Read the model definition and answer for the solid it produces. Units are mm, in the model's axes. A direction names the side the tool comes from. Coordinates: 2 decimals unless noted, no trailing zeros. Write each loop counter-clockwise with the first axis right and the second up, starting at its lowest first coordinate (ties: lowest second). Pieces come first, ordered by that corner, then holes.
1) The part is cut by section B-B (x = 0). Determine the outline of the cut face in (y, z), then the cut area to 3 significant figures.
2) The part is cut by section A-A (z = 0). Determine the outline of the cut face in (x, y), then the cut area to 3 significant figures.
3) Which of the six approach directions +Z, -Z, +X, -X, +Y, -Y give full straight-line access (tool end or side, diameter ignored) to faces 1 (the face through (1.172, 0.74, -8.923)), 2 (the face through (0, 5, 1))?
4) Each of these flat-tipped pins is pushed along its axis until it touches: pin 1 Ø3 at (x, z) = (-2, 4.5) entering from +Y; pin 2 Ø5 at (x, y) = (5.5, 3) entering from -Z; pin 3 Ø5 at (x, y) = (-5.5, 1.5) entering from +Z. Where does it stop, or does it pass through?
5) Find the intervals of material crossed by line 1 (Y direction, x = 0.5, z = -3); line 2 (Z direction, x = -0.25, y = 1.25); line 3 (X direction, y = 0.75, z = 8.25), in increasing order.
6) The part is cut by section C-C (y = 6). Determine the outline of the cut face in (x, z), then the cut area to 3 significant figures.
Autodesk Inventor part; units mm, degrees
ref_plane "YZ Plane" through (0, 0, 0) normal (1, 0, 0) x (0, 1, 0)
ref_plane "XZ Plane" through (0, 0, 0) normal (0, 1, 0) x (-1, 0, 0)
ref_plane "XY Plane" through (0, 0, 0) normal (0, 0, 1) x (1, 0, 0)
sketch "Boceto1" plane through (0, 0, 0) normal (0, 1, 0) x (-1, 0, 0)
  circle A0 centre (0, 0) radius 9
  circle A1 centre (0, 0) radius 1
  dimension "d0" = 18
extrude "Extrusión1" add sketch "Boceto1" along normal blind 2
extrude "Extrusión2" add sketch "Boceto1" along normal blind 9 contours A1
chamfer "Chaflán1" distance 0.5 angle 45 1 edges at (9, 2, 0)
fillet "Empalme1" radius 1 1 edges at (1, 9, 0)
properties part number "markers_base"
Reported:
1. outline: (0, -9) - (1.5, -9) - (2, -8.5) - (2, -1) - (8, -1) arc R1 ccw to (8, 1) - (2, 1) - (2, 8.5) - (1.5, 9) - (0, 9) - close
1. area: 49.3 mm2
2. outline: (-9, 0) - (9, 0) - (9, 1.5) - (8.5, 2) - (1, 2) - (1, 8) arc R1 ccw to (-1, 8) - (-1, 2) - (-8.5, 2) - (-9, 1.5) - close
2. area: 49.3 mm2
3. face 1: +Y, -Y
3. face 2: +Y
4. pin 1: stops at y = 2
4. pin 2: stops at z = -8.29
4. pin 3: stops at z = 8.49
5. line 1: y = 0 to 2
5. line 2: z = -9 to 9
5. line 3: x = -3.6 to 3.6
6. outline: circle Ø2 at (0, 0)
6. area: 3.14 mm2
